Can you work these out from the model? Positions are in its coordinate system, mm. A direction names the side the tool comes from. Give positions to 0.01 mm unless a question says otherwise; leave off trailing zeros. Order: outer loops, then holes, each group sorted by start corner. A loop starts at its lowest first (then second) coordinate and runs counter-clockwise, first axis right, second up. Notation, with made-up numbers: M 25.5,20.5 L 33.5,20.5 A5 ccw 33.5,29.5 Z; hole C 78.25,54 d7. An arc over 180 degrees is marked long. Use one line per item in the form item = value. Start each with the question number.
1. I want a section at A-A, the plane y = 0. List the corners of the cut face in (x, z) for me.
2. I want a section at C-C, the plane z = -141. List the corners of the cut face in (x, y) for me.
3. Will these pins go through, and if not, where does the flat tip stop? P1, Ø10, axis at x = 19.5, z = -116.5, coming from the +Y side; P2, Ø4, axis at y = 48, z = -46, coming from the +X side; P3, Ø1.5, axis at y = -50.5, z = 14.5, coming from the -X side.
4. I need wall thicknesses on L1, parallel to Z at x = 26, y = -60.5; L2, parallel to X at y = 1, z = -168.5; L3, parallel to Z at x = 23, y = -25. Which ranges of each line are inside material? Lowest first, please.
5. For faces 1 (the face through (0, 0, -398.018)), 2 (the face through (18, -18, -244.856)), which set-ups out of +Z, -Z, +X, -X, +Y, -Y let a thin tool reach every point of the face, with its end or its side?
6. I want a section at D-D, the plane x = 52. List the corners of the cut face in (y, z) for me, and give its area (3 significant figures).
```python
from build123d import *

# Parameters (mm, degrees)
F0_R          = 71.561005
F1_DEPTH      = 70.104
F2_R          = 65.314313
F3_DEPTH      = 62.23
F3_DEPTH_BACK = 119.126
F4_R          = 42.050536
F5_DEPTH      = 25.4
F5_DEPTH_BACK = 244.856
F6_R          = 23.371581
F7_DEPTH      = 25.4
F7_DEPTH_BACK = 398.018


with BuildPart() as f1:
    # F0 (on Top) → F1 (new body)
    with BuildSketch(Plane.XY):
        Circle(F0_R)
    extrude(amount=F1_DEPTH)

    # F2 (on Top) → F3 (join, two sides)
    with BuildSketch(Plane.XY) as f3_sk:
        Circle(F2_R)
    extrude(amount=F3_DEPTH)
    extrude(f3_sk.sketch, amount=-F3_DEPTH_BACK)

    # F4 (on Top) → F5 (join, two sides)
    with BuildSketch(Plane.XY) as f5_sk:
        Circle(F4_R)
    extrude(amount=F5_DEPTH)
    extrude(f5_sk.sketch, amount=-F5_DEPTH_BACK)

    # F6 (on Top) → F7 (join, two sides)
    with BuildSketch(Plane.XY) as f7_sk:
        Circle(F6_R)
    extrude(amount=F7_DEPTH)
    extrude(f7_sk.sketch, amount=-F7_DEPTH_BACK)


solid = f1.part
```
Check result:
q1.outline = M -71.56,0 L -65.31,0 L -65.31,-119.13 L -42.05,-119.13 L -42.05,-244.86 L -23.37,-244.86 L -23.37,-398.02 L 23.37,-398.02 L 23.37,-244.86 L 42.05,-244.86 L 42.05,-119.13 L 65.31,-119.13 L 65.31,0 L 71.56,0 L 71.56,70.1 L -71.56,70.1 Z
q2.outline = C 0,0 d84.1
q3.P1 = 63.68
q3.P2 = 46.37
q3.P3 = -51.44
q4.L1 = 0 to 70.1
q4.L2 = -42.04 to 42.04
q4.L3 = -244.86 to 70.1
q5.face_1 = -Z, +X, -X, +Y, -Y
q5.face_2 = -Z
q6.outline = M -49.16,0 L -39.52,0 L -39.52,-119.13 L 39.52,-119.13 L 39.52,0 L 49.16,0 L 49.16,70.1 L -49.16,70.1 Z
q6.area = 16,300 mm2
